```python
from build123d import *

# Parameters (mm, degrees)
BOSS_EXTRUDE1_DEPTH                       = 60
TAPPED_HOLE_FOR_M2_5X0_45_HELICOIL1_D     = 2.55
TAPPED_HOLE_FOR_M2_5X0_45_HELICOIL1_DEPTH = 4
TAPPED_HOLE_FOR_M2_5X0_45_HELICOIL1_TIP   = 0.766097289
F_1_2_1_2_DIAMETER_HOLE1_D                = 1.2
F_1_2_1_2_DIAMETER_HOLE1_DEPTH            = 6.45
F_1_2_1_2_DIAMETER_HOLE1_TIP              = 0.360516371


with BuildPart() as part:
    # Sketch1 → Boss-Extrude1 (new body)
    with BuildSketch(Plane(origin=(0, 0, 0), x_dir=(1, 0, 0), z_dir=(0, 1, 0))):
        with BuildLine():
            Line((-0.83484861, 0), (0.83484861, 0))
            ThreePointArc((0.83484861, 0), (2.790632181, 2.930008344), (5.641101056, 5))
            Line((5.641101056, 5), (5.641101056, 6))
            Line((5.641101056, 6), (-5.641101056, 6))
            Line((-5.641101056, 6), (-5.641101056, 5))
            ThreePointArc((-5.641101056, 5), (-2.790632181, 2.930008344), (-0.83484861, 0))
        make_face()
    extrude(amount=BOSS_EXTRUDE1_DEPTH)

    # Tapped Hole for M2.5x0.45 Helicoil1
    with Locations(Plane(origin=(0, 30, -6), x_dir=(-1, 0, 0), z_dir=(0, 0, -1))):
        with Locations((0, 0)):
            Hole(TAPPED_HOLE_FOR_M2_5X0_45_HELICOIL1_D / 2, depth=TAPPED_HOLE_FOR_M2_5X0_45_HELICOIL1_DEPTH)
            with Locations((0, 0, -(TAPPED_HOLE_FOR_M2_5X0_45_HELICOIL1_DEPTH + TAPPED_HOLE_FOR_M2_5X0_45_HELICOIL1_TIP / 2))):  # 118° drill point
                Cone(0, TAPPED_HOLE_FOR_M2_5X0_45_HELICOIL1_D / 2, TAPPED_HOLE_FOR_M2_5X0_45_HELICOIL1_TIP, mode=Mode.SUBTRACT)

    # Ø1.2 (1.2) Diameter Hole1
    with Locations(Plane(origin=(0, 30, -6), x_dir=(-1, 0, 0), z_dir=(0, 0, -1))):
        with Locations((0, 0)):
            Hole(F_1_2_1_2_DIAMETER_HOLE1_D / 2, depth=F_1_2_1_2_DIAMETER_HOLE1_DEPTH)
            with Locations((0, 0, -(F_1_2_1_2_DIAMETER_HOLE1_DEPTH + F_1_2_1_2_DIAMETER_HOLE1_TIP / 2))):  # 118° drill point
                Cone(0, F_1_2_1_2_DIAMETER_HOLE1_D / 2, F_1_2_1_2_DIAMETER_HOLE1_TIP, mode=Mode.SUBTRACT)


solid = part.part
```
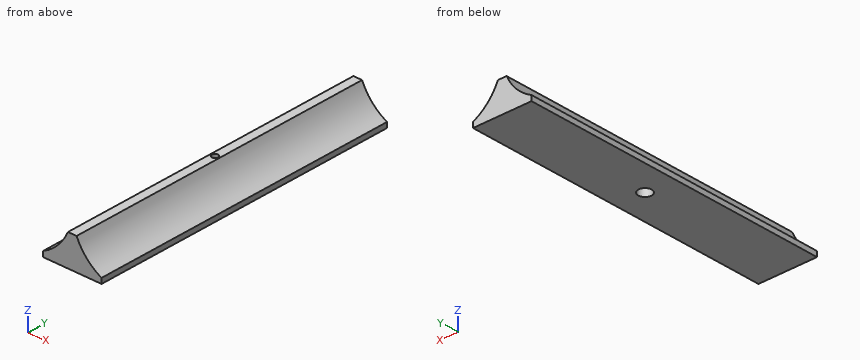
Input: part model. Units: mm. Frame: model coordinates. Coordinates: 2 decimals unless noted, no trailing zeros. Write each loop counter-clockwise with the first axis right and the second up, starting at its lowest first coordinate (ties: lowest second). Pieces come first, ordered by that corner, then holes. Notation, with made-up numbers: (-13.5, 81) - (14.5, 81) arc R28 cw to (14.5, 119) - close; hole circle Ø2 at (45, 30.5). An arc over 180 degrees is marked (long way). Put each result on its own line as item: value. Start each with the question number.
1) Cut plane A-A (x = 0). Return the cut outline in (y, z) (3 decimals), plus the area to 3 significant figures.
2) Contact query for flat-ended pins moving along their axis: pin 1 (1.6 mm diameter, centred on x = 0, y = 30, fed in from -Z); pin 2 (1 mm diameter, centred on x = 4.5, y = 36, fed in from +Z); pin 3 (2 mm diameter, centred on x = 4.5, z = -3, fed in from -Y). Output: stop coordinate, or through.
3) Cut plane D-D (z = -3.75). Return the cut outline in (x, y) (3 decimals).
4) Cut plane B-B (y = 30). Return the cut outline in (x, z) (3 decimals).
5) Cut plane C-C (y = 37.5). Return the cut outline in (x, z).
6) Ray query, L1, parallel to Y at x = 0, z = -1.1; L2, parallel to Y at x = 0, z = -5.1 (3 decimals); L3, parallel to Z at x = -2, y = 26. Return the intervals inside material, ascending.
Resolved:
1. outline: (0, -6) - (28.725, -6) - (28.725, -2) - (29.4, -1.594) - (29.4, 0) - (0, 0) - close; (30.6, -1.594) - (31.275, -2) - (31.275, -6) - (60, -6) - (60, 0) - (30.6, 0) - close
1. area: 347 mm2
2. pin 1: stops at z = -1.71
2. pin 2: stops at z = -4
2. pin 3: passes through
3. outline: (-3.68, 0) - (3.68, 0) - (3.68, 60) - (-3.68, 60) - close; hole circle Ø2.55 at (0, 30)
4. outline: (-5.641, -6) - (-1.275, -6) - (-1.275, -2) - (-0.6, -1.594) - (-0.6, 0) - (-0.835, 0) arc R10 cw to (-5.641, -5) - close; (0.6, -1.594) - (1.275, -2) - (1.275, -6) - (5.641, -6) - (5.641, -5) arc R10 cw to (0.835, 0) - (0.6, 0) - close
5. outline: (-5.64, -6) - (5.64, -6) - (5.64, -5) arc R10 cw to (0.83, 0) - (-0.83, 0) arc R10 cw to (-5.64, -5) - close
6. L1: y = 0 to 29.4, 30.6 to 60
6. L2: y = 0 to 28.725, 31.275 to 60
6. L3: z = -6 to -2
